Input: part model. Units: mm. Frame: model coordinates. Coordinates: 2 decimals unless noted, no trailing zeros. Order: outer loops, then holes, each group sorted by start corner. A loop starts at its lowest first (then second) coordinate and runs counter-clockwise, first axis right, second up. Notation, with made-up numbers: (6.25, 86) - (36.25, 86) arc R15 ccw to (36.25, 109) - close; hole circle Ø2 at (53, -29). An arc over 180 degrees is marked (long way). Answer as CSV lines item,"result". Start each with the question number.
Item 1: Section B-B (y = 391). Output: boundary loops of the cut face in (x, z).
Item 2: Section A-A (x = 1.8). Output: boundary loops of the cut face in (y, z), and give its area (3 significant figures).
Item 3: First-contact query: pin 1 (1.5 mm diameter, centred on x = 1, z = 241.5, fed in from -Y); pin 2 (1.5 mm diameter, centred on x = 0.5, y = 292, fed in from -Z). Flat tips, straight axial feed; report the tip coordinate or a pass-through.
Item 4: Section C-C (z = -75). Output: boundary loops of the cut face in (x, y), and give its area (3 significant figures).
Item 5: Material intervals for line 1 along Z through (x, y) = (0.55, 308); line 2 along Z through (x, y) = (1.75, 513.5), sorted ascending.
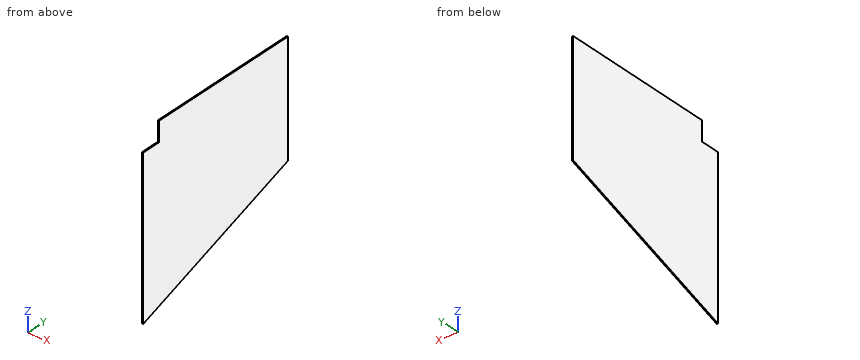
from build123d import *

# Parameters (mm, degrees)
BOSS_EXTRUDE1_DEPTH = 3
SKETCH2_W           = 50
SKETCH2_H           = 50
CUT_EXTRUDE1_DEPTH  = 10


with BuildPart() as part:
    # Sketch1 → Boss-Extrude1 (new body)
    with BuildSketch(Plane(origin=(0, 0, 0), x_dir=(0, 0, -1), z_dir=(1, 0, 0))):
        Polygon((31.669668796, 625.573683549), (191.669668796, 173.025343589), (-258.330331204, 173.025343589), (-258.330331204, 625.573683549), align=None)
    extrude(amount=BOSS_EXTRUDE1_DEPTH)

    # Sketch2 → Cut-Extrude1 (cut)
    with BuildSketch(Plane.ZY):
        with Locations((233.330331204, 198.025343589)):
            Rectangle(SKETCH2_W, SKETCH2_H)
    extrude(amount=-CUT_EXTRUDE1_DEPTH, mode=Mode.SUBTRACT)


solid = part.part
Determined:
1,outline,"(0, -114.6) - (3, -114.6) - (3, 258.33) - (0, 258.33) - close"
2,outline,"(173.03, -191.67) - (625.57, -31.67) - (625.57, 258.33) - (223.03, 258.33) - (223.03, 208.33) - (173.03, 208.33) - close"
2,area,"165,000 mm^2"
3,pin 1,"stops at y = 223.03"
3,pin 2,"stops at z = -149.87"
4,outline,"(0, 173.03) - (3, 173.03) - (3, 503.02) - (0, 503.02) - close"
4,area,"990 mm^2"
5,line 1,"z = -143.95 to 258.33"
5,line 2,"z = -71.29 to 258.33"
